from build123d import *

# Parameters (mm, degrees)
SKETCH1_W                  = 5.5
SKETCH1_H                  = 6.24
EXTRUDE1_DEPTH             = 5
SKETCH6_W                  = 9.5
SKETCH6_H                  = 14
EXTRUDE2_DEPTH             = 5.23
F_3_7_3_7_DIAMETER_HOLE1_D = 3.7
SKETCH3_R                  = 1.25
CUT_EXTRUDE1_DEPTH         = 7.24
CHAMFER2_SIZE              = 0.5
SKETCH8_W                  = 9.5
SKETCH8_H                  = 1
EXTRUDE4_DEPTH             = 7.24


with BuildPart() as part:
    # Sketch1 → Extrude1 (new body, symmetric)
    with BuildSketch(Plane.XY):
        Rectangle(SKETCH1_W, SKETCH1_H)
    extrude(amount=EXTRUDE1_DEPTH, both=True)

    # Sketch6 → Extrude2 (add)
    with BuildSketch(Plane(origin=(0, 3.12, 0), x_dir=(1, 0, 0), z_dir=(0, 1, 0))):
        Rectangle(SKETCH6_W, SKETCH6_H)
    extrude(amount=-EXTRUDE2_DEPTH)

    # 3.7 _3.7_ Diameter Hole1 (through all)
    with Locations(Plane(origin=(0.72811331, -3.12, 5.297514906), x_dir=(1, 0, 0), z_dir=(0, -1, 0))):
        with Locations((-0.72811331, -7.797514906)):
            Hole(F_3_7_3_7_DIAMETER_HOLE1_D / 2)

    # Sketch3 → Cut-Extrude1 (cut, through all)
    with BuildSketch(Plane(origin=(0, -3.12, 0), x_dir=(-1, 0, 0), z_dir=(0, -1, 0))):
        with Locations(Location((0, -2.5, 0), (0, 0, 180))):  # turned: the seam where the file's is
            Circle(SKETCH3_R)
    extrude(amount=-CUT_EXTRUDE1_DEPTH, mode=Mode.SUBTRACT)

    # Chamfer2
    chamfer2_edges = [part.edges().sort_by_distance(p)[0] for p in [
        (4.75, 0.505, 7),
        (-4.75, 0.505, 7),
    ]]
    chamfer(chamfer2_edges, length=CHAMFER2_SIZE)

    # Sketch8 → Extrude4 (cut, through all)
    with BuildSketch(Plane.XZ.offset(3.12)):
        with Locations((0, -6.5)):
            Rectangle(SKETCH8_W, SKETCH8_H)
    extrude(amount=-EXTRUDE4_DEPTH, mode=Mode.SUBTRACT)


solid = part.part
Input: part model. Units: mm. Frame: model coordinates. A direction names the side the tool comes from. Give positions to 0.01 mm unless a question says otherwise; leave off trailing zeros. Write each loop counter-clockwise with the first axis right and the second up, starting at its lowest first coordinate (ties: lowest second). Pieces come first, ordered by that corner, then holes. Notation, with made-up numbers: (27.25, 11) -> (77.25, 11) arc R20 ccw to (77.25, 16) -> close; hole circle Ø6 at (5, 24). An arc over 180 degrees is marked (long way). Use one line per item in the form item = value. Start each with the question number.
1) Section query A-A on z = -2.5. Return the cut outline in (x, y).
2) Section query D-D on z = -0.5. Return the cut outline in (x, y), then the cut area to 3 significant figures.
3) Ray query, probe 1 along Z at (x, y) = (0, 1.75); probe 2 along Z at (x, y) = (-0.5, 2.5); probe 3 along Y at (x, z) = (-2.75, 5.25). Return the intervals inside material, ascending. Write a range as from..to.
4) Section query C-C on x = 0. Return the cut outline in (y, z).
5) Set-up query: faces 1 (the flat face through (-2.75, -2.6, 0.1)), 2 (the flat face through (0, -2.6, -5)), 3 (the flat face through (2.75, -2.6, 0.1)). Return all of +Z, -Z, +X, -X, +Y, -Y with unobstructed straight access to the full face (end or side cutting, diameter ignored); none if empty.
6) Section query B-B on y = 2.5. Return the cut outline in (x, z), then the cut area to 3 significant figures.
7) Pin query (flat end, axial travel): pin 1 (1.1 mm diameter, centred on x = -1, y = -3, fed in from -Z); pin 2 (0.5 mm diameter, centred on y = -2.5, z = 0.5, fed in from +X). Return the tip coordinate at first contact, or that it passes through.
Outcome:
q1.outline = (-4.75, -2.11) -> (-2.75, -2.11) -> (-2.75, -3.12) -> (-1.85, -3.12) -> (-1.85, 3.12) -> (-4.75, 3.12) -> close; (1.85, -3.12) -> (2.75, -3.12) -> (2.75, -2.11) -> (4.75, -2.11) -> (4.75, 3.12) -> (1.85, 3.12) -> close
q2.outline = (-4.75, -2.11) -> (-2.75, -2.11) -> (-2.75, -3.12) -> (2.75, -3.12) -> (2.75, -2.11) -> (4.75, -2.11) -> (4.75, 3.12) -> (-4.75, 3.12) -> close
q2.area = 55.2 mm^2
q3.probe_1 = -6..-4.35, -0.65..1.25, 3.75..7
q3.probe_2 = -6..-4.28, -0.72..1.35, 3.65..7
q3.probe_3 = -2.11..3.12
q4.outline = (-3.12, -5) -> (-2.11, -5) -> (-2.11, -6) -> (3.12, -6) -> (3.12, -4.35) -> (-3.12, -4.35) -> close; (-3.12, -0.65) -> (3.12, -0.65) -> (3.12, 1.25) -> (-3.12, 1.25) -> close; (-3.12, 3.75) -> (3.12, 3.75) -> (3.12, 7) -> (-2.11, 7) -> (-2.11, 5) -> (-3.12, 5) -> close
q5.face_1 = +Z, -Z, -X, -Y
q5.face_2 = -Z, +X, -X, -Y
q5.face_3 = +Z, -Z, +X, -Y
q6.outline = (-4.75, -6) -> (4.75, -6) -> (4.75, 6.5) -> (4.25, 7) -> (-4.25, 7) -> (-4.75, 6.5) -> close; hole circle Ø3.7 at (0, -2.5); hole circle Ø2.5 at (0, 2.5)
q6.area = 108 mm^2
q7.pin_1 = -5
q7.pin_2 = 2.75
